For this review, take the finished solid that the model builds, in its own axes (mm). A direction names the side the tool comes from. Give positions to 0.01 mm unless a question says otherwise; leave off trailing zeros. Loops run counter-clockwise (first coordinate to the right, second up) from the corner with the lowest first, then second, coordinate; pieces in that order, holes last. Notation, with made-up numbers: (67.25, -5) - (83.25, -5) arc R21 ccw to (83.25, 3) - close; hole circle Ø4 at (85, 3). An arc over 180 degrees is marked (long way). Put each result on its own line as item: value. Start each with the question number.
from build123d import *

# Parameters (mm, degrees)
CROQUIS1_W              = 220
CROQUIS1_H              = 143
SALIENTE_EXTRUIR1_DEPTH = 5
CROQUIS2_W              = 210
CROQUIS2_H              = 133
CORTAR_EXTRUIR1_DEPTH   = 3
CROQUIS3_W              = 220
CROQUIS3_H              = 157.6
SALIENTE_EXTRUIR2_DEPTH = 3
CROQUIS4_W              = 5.2
CROQUIS4_H              = 20
CORTAR_EXTRUIR2_DEPTH   = 136.548662848


with BuildPart() as part:
    # Croquis1 → Saliente-Extruir1 (new body)
    with BuildSketch(Plane.XY):
        Rectangle(CROQUIS1_W, CROQUIS1_H)
    extrude(amount=SALIENTE_EXTRUIR1_DEPTH)

    # Croquis2 → Cortar-Extruir1 (cut)
    with BuildSketch(Plane.XY.offset(5)):
        Rectangle(CROQUIS2_W, CROQUIS2_H)
    extrude(amount=-CORTAR_EXTRUIR1_DEPTH, mode=Mode.SUBTRACT)

    # Croquis3 → Saliente-Extruir2 (add)
    with BuildSketch(Plane(origin=(0, 0, 0), x_dir=(-1, 0, 0), z_dir=(0, 0, -1))):
        Rectangle(CROQUIS3_W, CROQUIS3_H)
    extrude(amount=SALIENTE_EXTRUIR2_DEPTH)

    # Croquis4 → Cortar-Extruir2 (cut, through all)
    with BuildSketch(Plane(origin=(0, 0, -3), x_dir=(-1, 0, 0), z_dir=(0, 0, -1))):
        with Locations((-107.4, 68.8)):
            Rectangle(CROQUIS4_W, CROQUIS4_H)
        with Locations((-107.4, -68.8)):
            Rectangle(CROQUIS4_W, CROQUIS4_H)
    extrude(amount=-CORTAR_EXTRUIR2_DEPTH, mode=Mode.SUBTRACT)


solid = part.part
1) Machinability: for faces 1 (the flat face through (-4, -71.5, 2)), 2 (the flat face through (-1, 75, 0)), 3 (the flat face through (107, 58.8, 1)), 4 (the flat face through (2, 1, -3)), 5 (the flat face through (-110, -1, 1)), which of the approach directions +Z, -Z, +X, -X, +Y, -Y give a long, thin tool a straight path to every point of the face, cutting with its end or side? Answer none if there is none.
2) Take a section at B-B on x = -31. State the section outline as (y, z) points.
3) Mouldability with a two-part tool opening along X and no side actions: class faces 6 (the flat face through (107, -58.8, 1)), 7 (the flat face through (104.8, -69, 0)), 8 (the flat face through (-1, 1, 2)) as released by +X, released by -X, zero draft, split by the parting line, or undercut.
4) Take a section at A-A on z = 3.25. State the section outline as (x, y) points, and give its area (3 significant figures).
5) Wall thickness on probe 1 along X at (y, z) = (-34.5, 3.25); probe 2 along Y at (x, z) = (-86, 3.75); probe 3 along Y at (x, z) = (-38.5, 1.75): over which ranges is each line inside the solid? List them lowest first.
6) Insertion check: P1, Ø1.5, axis at x = -7.5, z = 4, coming from the +Y side; P2, Ø2.5, axis at x = -31, z = 2, coming from the -Y side; P3, Ø4, axis at x = 107.5, z = -0.5, coming from the -Y side. Each pin has a flat end and moves straight along its axis. Give the tip position at first contact, or say it passes through.
7) Take a section at C-C on y = -17. State the section outline as (x, z) points, and give its area (3 significant figures).
Answers follow:
1. face 1: +Z, +X, -X, -Y
1. face 2: +Z, +X, -X, +Y
1. face 3: +Z, -Z, +X, +Y
1. face 4: -Z, +X, -X, +Y, -Y
1. face 5: +Z, -Z, -X, +Y, -Y
2. outline: (-78.8, -3) - (78.8, -3) - (78.8, 0) - (71.5, 0) - (71.5, 5) - (66.5, 5) - (66.5, 2) - (-66.5, 2) - (-66.5, 5) - (-71.5, 5) - (-71.5, 0) - (-78.8, 0) - close
3. face 6: zero draft
3. face 7: released by +X
3. face 8: undercut
4. outline: (-110, -71.5) - (104.8, -71.5) - (104.8, -66.5) - (-105, -66.5) - (-105, 66.5) - (104.8, 66.5) - (104.8, 71.5) - (-110, 71.5) - close; (105, -58.8) - (110, -58.8) - (110, 58.8) - (105, 58.8) - close
4. area: 3,400 mm2
5. probe 1: -110 to -105, 105 to 110
5. probe 2: -71.5 to -66.5, 66.5 to 71.5
5. probe 3: -71.5 to 71.5
6. P1: y = 71.5
6. P2: y = -71.5
6. P3: y = -58.8
7. outline: (-110, -3) - (110, -3) - (110, 5) - (105, 5) - (105, 2) - (-105, 2) - (-105, 5) - (-110, 5) - close
7. area: 1,130 mm2
